Solid Edge part; units mm, degrees
sketch "Sketch1" plane through (0, 0, 0) normal (0, 0, 1) x (1, 0, 0)
  line L0 (-45, -8) -> (-35, -8)
  line L1 (-35, -8) -> (-28.3333, 0)
  line L2 (-28.3333, 0) -> (0, 0)
  line L3 (0, 0) -> (0, 10)
  line L4 (0, 10) -> (-30, 10)
  line L5 (-30, 10) -> (-45, -8)
  dimension "D1" = 35
  dimension "D2" = 30
  dimension "D3" = 45
extrude "Protrusion1" add sketch "Sketch1" along normal mid plane 18
sketch "Sketch2" plane through (-35, 0, 0) normal (1, 0, 0) x (0, 1, 0)
  circle A0 centre (-21, 0) radius 16
  dimension "D1" = 21
extrude "Protrusion2" add sketch "Sketch2" against normal up to vertex (10 mm away)
hole "Hole_1" at (-35, -12.25, 0) direction (-1, 0, 0) diameter 3.6 end up to next countersink diameter 6.94 countersink angle 90
hole "Hole1" at (-35, -21, -8.75) direction (-1, 0, 0) diameter 3.6 end up to next countersink diameter 6.94 countersink angle 90
hole "Hole2" at (-35, -29.75, 0) direction (-1, 0, 0) diameter 3.6 end up to next countersink diameter 6.94 countersink angle 90
hole "Hole3" at (-35, -21, 8.75) direction (-1, 0, 0) diameter 3.6 end up to next countersink diameter 6.94 countersink angle 90
mirror "Mirror1" about plane through (0, 0, 0) normal (1, 0, 0) of "Protrusion2", "Protrusion1", "Hole_1", "Hole1", "Hole2", "Hole3"
sketch "Sketch3" plane through (0, 0, 0) normal (0, 0, 1) x (1, 0, 0)
  line L0 (45, -35) -> (42, -37)
  line L1 (42, -37) -> (42, -40)
  line L2 (42, -40) -> (45, -40)
  line L3 (45, -40) -> (45, -35)
  dimension "D1" = 42
  dimension "D2" = 45
  dimension "D3" = 42
revolve "RevolvedCutout1" cut sketch "Sketch3" angle 360 about axis through (45, -21, 0) along (-1, 0, 0)
mirror "Mirror2" about plane through (0, 0, 0) normal (1, 0, 0) of "RevolvedCutout1"
hole "Hole_5" at (20, 5, -9) direction (0, 0, 1) diameter 3.4 end up to next start chamfer 0.3 start chamfer angle 45 end chamfer 0.3 end chamfer angle 45
hole "Hole4" at (-20, 5, -9) direction (0, 0, 1) diameter 3.4 end up to next start chamfer 0.3 start chamfer angle 45 end chamfer 0.3 end chamfer angle 45
hole "Hole_7" at (10, 10, 0) direction (0, -1, 0) diameter 2.8 depth 30 tip angle 118 start chamfer 0.3 start chamfer angle 45 end chamfer 0.3 end chamfer angle 45
hole "Hole5" at (-10, 10, 0) direction (0, -1, 0) diameter 2.8 depth 30 tip angle 118 start chamfer 0.3 start chamfer angle 45 end chamfer 0.3 end chamfer angle 45
properties material "Polyethylene, low density"
Check sheet for the modelled part. Datum: model origin and axes. Units: mm. A direction names the side the tool comes from. Round coordinates to 2 decimals unless told otherwise and drop trailing zeros. Loops run counter-clockwise (first coordinate to the right, second up) from the corner with the lowest first, then second, coordinate; pieces in that order, holes last. Notation, with made-up numbers: (-23.75, 78) - (11.25, 78) arc R29 ccw to (11.25, 112) - close; hole circle Ø4 at (41, 82). An arc over 180 degrees is marked (long way). Answer as CSV lines item,"result". Start each with the question number.
Item 1: Depth check by flat-ended pin: P1, Ø14.5, axis at x = -5, y = 2, coming from the +Z side; P2, Ø5.5, axis at x = -11.5, y = 1.5, coming from the -Z side; P3, Ø5, axis at y = -7.5, z = -10, coming from the +X side. Enter the tip coordinate at first touch or a pass-through.
Item 2: Section check A-A (y = 5). Record the boundary of the cut face in (x, z).
Item 3: Set-up check for faces 1 (the flat face through (45, -21, 0)), 2 (the flat face through (-42, -4.6, 0.1)), 3 (the flat face through (-1, 3, 9)): record each of +Z, -Z, +X, -X, +Y, -Y from which the full face is reachable in a straight line by a thin tool's end or side.
Item 4: Section check C-C (y = -21). Count the separate pieces of the cut face and the enclosed holes in it, and give its area (3 significant figures).
Item 5: Scan lines: line 1 (X direction, y = -15.5, z = -4); line 2 (Y direction, x = 41, z = 0); line 3 (X direction, y = 7, z = 0). Record each from-to range of solid material in increasing order. Write a range as [from, to].
Item 6: Release check for a two-part mould opening along X. For faces 4 (the flat face through (0, 10, 0)), 5 (the flat face through (42, -4.6, 0.1)), 6 (the cylindrical face through (11.367, 4.934, -0.303)) record: +X half, -X half, draft (parallel to the pull), parting line (faces both ways), or undercut.
Item 7: Section check B-B (x = 10). Record the boundary of the cut face in (y, z), and give its area (3 significant figures).
Report:
1,P1,"stops at z = 9"
1,P2,"stops at z = -9"
1,P3,"stops at x = 44.55"
2,outline,"(-34.17, -9) - (-22, -9) - (-21.7, -8.7) - (-21.7, 8.7) - (-22, 9) - (-34.17, 9) - close; (-18.3, -8.7) - (-18, -9) - (18, -9) - (18.3, -8.7) - (18.3, 8.7) - (18, 9) - (-18, 9) - (-18.3, 8.7) - close; (21.7, -8.7) - (22, -9) - (34.17, -9) - (34.17, 9) - (22, 9) - (21.7, 8.7) - close; hole circle Ø2.8 at (-10, 0); hole circle Ø2.8 at (10, 0)"
3,face 1,"+Z, -Z, +X, +Y, -Y"
3,face 2,"-X, +Y"
3,face 3,"+Z, +X, -X, +Y"
4,separate pieces,"6"
4,enclosed holes,"0"
4,area,"473 mm2"
5,line 1,"x = [-45, -35], [35, 45]"
5,line 2,"y = [-37, -31.55], [-27.95, -14.05], [-10.45, -3.2]"
5,line 3,"x = [-32.5, -11.4], [-8.6, 8.6], [11.4, 32.5]"
6,face 4,"draft"
6,face 5,"+X half"
6,face 6,"undercut"
7,outline,"(0, -9) - (10, -9) - (10, -1.7) - (9.7, -1.4) - (0.3, -1.4) - (0, -1.7) - close; (0, 1.7) - (0.3, 1.4) - (9.7, 1.4) - (10, 1.7) - (10, 9) - (0, 9) - close"
7,area,"152 mm2"
